Work out the finished part from the listing and answer in its coordinate system (mm). Face numbers are marked on the shaded views. Coordinates: 2 decimals unless noted, no trailing zeros. Loops run counter-clockwise (first coordinate to the right, second up) from the corner with the lowest first, then second, coordinate; pieces in that order, holes last. Notation, with made-up numbers: (44.25, 4) -> (72.25, 4) arc R32 ccw to (72.25, 39) -> close; hole circle Ø7 at (-29.5, -28.5). An arc over 180 degrees is marked (long way). Use a Markdown table: item, result.
from build123d import *

# Parameters (mm, degrees)
SKETCH1_R           = 3.81
BOSS_EXTRUDE1_DEPTH = 38.1
SKETCH2_R           = 6.35
BOSS_EXTRUDE2_DEPTH = 6.35
SKETCH6_R           = 2.8575
BOSS_EXTRUDE3_DEPTH = 2.54
SKETCH14_W          = 3.81
SKETCH14_H          = 3.81
CUT_EXTRUDE1_DEPTH  = 38.1
BOSS_EXTRUDE5_START = -25.4
BOSS_EXTRUDE5_DEPTH = 25.4
SKETCH16_R          = 1.5875
CUT_EXTRUDE2_DEPTH  = 25.4


# Read off the part's stored shape, not the designer's step: Boss-Extrude5
with BuildPart() as part:
    # Sketch1 → Boss-Extrude1 (new body)
    with BuildSketch(Plane.XY):
        with Locations(Location((0, 0, 0), (0, 0, 180))):
            Circle(SKETCH1_R)
    extrude(amount=BOSS_EXTRUDE1_DEPTH)

    # Sketch2 → Boss-Extrude2 (add)
    with BuildSketch(Plane(origin=(0, 0, 0), x_dir=(-1, 0, 0), z_dir=(0, 0, -1))):
        Circle(SKETCH2_R)
    extrude(amount=BOSS_EXTRUDE2_DEPTH)

    # Sketch6 → Boss-Extrude3 (add)
    with BuildSketch(Plane.XY.offset(38.1)):
        Circle(SKETCH6_R)
    extrude(amount=-BOSS_EXTRUDE3_DEPTH)

    # Sketch14 → Cut-Extrude1 (cut)
    with BuildSketch(Plane.XY.offset(38.1)):
        Rectangle(SKETCH14_W, SKETCH14_H)
    extrude(amount=-CUT_EXTRUDE1_DEPTH, mode=Mode.SUBTRACT)

    # Boss-Extrude5 outline → Boss-Extrude5 (add)
    with BuildSketch(Plane.XY.offset(38.1).offset(BOSS_EXTRUDE5_START)):
        with BuildLine():
            ThreePointArc((-3.298088459, 1.907540961), (-1.903729096, 3.300290219), (0, 3.81))
            Line((0, 3.81), (-2.010168305, 4.316182263))
            ThreePointArc((-2.010168305, 4.316182263), (-2.380206411, 4.123596348), (-2.731973317, 3.899369726))
            Line((-2.731973317, 3.899369726), (-3.298088459, 1.907540961))
        make_face()
        with BuildLine():
            Line((2.011093908, 4.31641534), (0, 3.81))
            ThreePointArc((0, 3.81), (3.809999869, 0.001000002), (0.002000005, -3.809999475))
            Line((0.002000005, -3.809999475), (2.011795704, -4.316088438))
            ThreePointArc((2.011795704, -4.316088438), (2.38208523, -4.123386397), (2.734078384, -3.899000058))
            Line((2.734078384, -3.899000058), (3.301056788, -1.904133975))
            Line((3.301056788, -1.904133975), (4.744240085, -0.416644057))
            ThreePointArc((4.744240085, -0.416644057), (4.762499984, 0.000387099), (4.744172292, 0.417415282))
            Line((4.744172292, 0.417415282), (3.300056788, 1.905866025))
            Line((3.300056788, 1.905866025), (2.73344438, 3.899444381))
            ThreePointArc((2.73344438, 3.899444381), (2.381414754, 4.123773496), (2.011093908, 4.31641534))
        make_face()
        with BuildLine():
            Line((-2.009093908, -4.31641534), (0.002000005, -3.809999475))
            ThreePointArc((0.002000005, -3.809999475), (-1.901999931, -3.301287062), (-3.29709076, -1.909264917))
            Line((-3.29709076, -1.909264917), (-2.73144438, -3.899444381))
            ThreePointArc((-2.73144438, -3.899444381), (-2.379414754, -4.123773496), (-2.009093908, -4.31641534))
        make_face()
        with BuildLine():
            ThreePointArc((-3.300524979, -1.90332206), (-3.80999987, -0.000996951), (-3.3015206, 1.901594523))
            Line((-3.3015206, 1.901594523), (-4.742240085, 0.416644057))
            ThreePointArc((-4.742240085, 0.416644057), (-4.760499984, -0.000387099), (-4.742172292, -0.417415282))
            Line((-4.742172292, -0.417415282), (-3.300524979, -1.90332206))
        make_face()
    extrude(amount=BOSS_EXTRUDE5_DEPTH)

    # Sketch16 → Cut-Extrude2 (cut)
    with BuildSketch(Plane(origin=(-1.905, 0, 0), x_dir=(0, 0, -1), z_dir=(1, 0, 0))):
        with Locations(Location((-3.175, 0, 0), (0, 0, 90))):
            Circle(SKETCH16_R)
    extrude(amount=-CUT_EXTRUDE2_DEPTH, mode=Mode.SUBTRACT)


solid = part.part
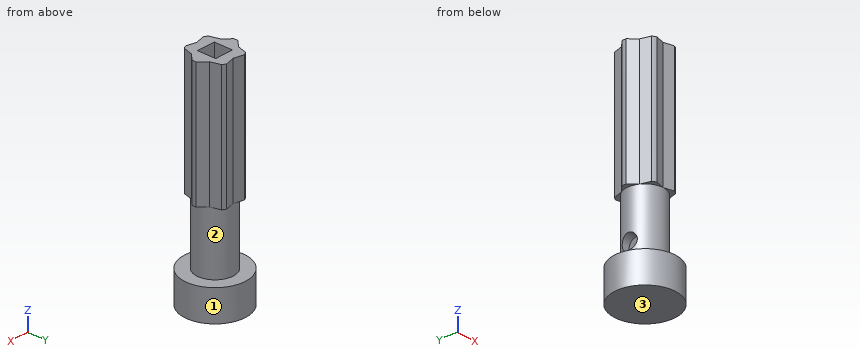
Q1. Section D-D on y = 3 is taken. Determine the outline of the cut face in (x, z).
Solved:
| item | result |
|---|---|
| outline | (-5.6, -6.35) -> (5.6, -6.35) -> (5.6, 0) -> (2.35, 0) -> (2.35, 12.7) -> (2.99, 12.7) -> (2.99, 38.1) -> (-2.99, 38.1) -> (-2.99, 12.7) -> (-2.35, 12.7) -> (-2.35, 0) -> (-5.6, 0) -> close |
Q2. Given pin 1 Ø5 at (y, z) = (2.5, 30) entering from -X; pin 2 Ø1.5 at (y, z) = (4, 18.5) entering from +X; pin 3 Ø1 at (y, z) = (4, 5.5) entering from -X, each flat-ended and moving along its own axis, determine where each tip first touches the part or whether it passes through.
Solved:
| item | result |
|---|---|
| pin 1 | x = -4.76 |
| pin 2 | x = 2.92 |
| pin 3 | x = -1.51 |
Q3. Determine the mould class of the marked faces 1, 2 and 3 for opening direction Z: pulls with the +Z half, pulls with the -Z half, needs draft (parallel to the pull), parting line crosses it, or undercut.
Solved:
| item | result |
|---|---|
| face 1 | needs draft |
| face 2 | undercut |
| face 3 | pulls with the -Z half |
Q4. Section C-C on x = 4.25 is taken. Determine the outline of the cut face in (y, z), and give its area (3 significant figures).
Solved:
| item | result |
|---|---|
| outline | (-4.72, -6.35) -> (4.72, -6.35) -> (4.72, 0) -> (-4.72, 0) -> close; (-0.93, 12.7) -> (0.93, 12.7) -> (0.93, 38.1) -> (-0.93, 38.1) -> close |
| area | 107 mm² |
Q5. Consider line 1 (Z direction, x = -2.6, y = 0); line 2 (Y direction, x = 2, z = 32.5); line 3 (X direction, y = 1.75, z = 4) (3 decimals). Determine where each line is inside the solid, lowest interval first. Write a range as [from, to].
Solved:
| item | result |
|---|---|
| line 1 | [-6.35, 1.59], [4.76, 38.1] |
| line 2 | [-4.31, 4.31] |
| line 3 | [-3.384, -1.905], [1.905, 3.384] |
